Could you check a few things on this model? Use its own coordinates, in mm. Face numbers are marked on the shaded views. Give positions to 0.01 mm unless a question says otherwise; leave off trailing zeros. Order: outer loops, then holes, each group sorted by start corner. A loop starts at its lowest first (then second) coordinate and runs counter-clockwise, first axis right, second up. Notation, with made-up numbers: (18.5, -34) -> (53.5, -34) arc R26 ccw to (53.5, -9) -> close; hole circle Ø3 at (64, 29). An arc over 180 degrees is marked (long way). Write each question's results on one line, items separated by ' | '.
Autodesk Inventor part; units mm, degrees
ref_plane "YZ Plane" through (0, 0, 0) normal (1, 0, 0) x (0, 1, 0)
ref_plane "XZ Plane" through (0, 0, 0) normal (0, 1, 0) x (-1, 0, 0)
ref_plane "XY Plane" through (0, 0, 0) normal (0, 0, 1) x (1, 0, 0)
sketch "Sketch1" plane through (0, 0, 0) normal (0, 0, 1) x (1, 0, 0)
  circle A0 centre (0, 0) radius 30
  circle A1 centre (0, 0) radius 24.5
  dimension "d0" = 49
  dimension "d1" = 60
extrude "Extrusion1" add sketch "Sketch1" against normal blind 1.1
sketch "Sketch2" plane through (0, 0, 0) normal (0, 0, 1) x (1, 0, 0)
  line L0 (0, 0) -> (0, 30) construction
  circle A0 centre (0, 0) radius 30 construction
  line L1 (-1.7914, 26.2382) -> (1.7914, 26.2382)
  line L2 (1.7914, 26.2382) -> (1.7914, 29.0379)
  line L3 (1.7914, 29.0379) -> (-1.7914, 29.0379)
  line L4 (-1.7914, 29.0379) -> (-1.7914, 26.2382)
  line L5 (-1.7914, 26.2382) -> (1.7914, 29.0379) construction
  line L6 (1.7914, 26.2382) -> (-1.7914, 29.0379) construction
  point P0 (0, 27.6381)
extrude "Extrusion2" add sketch "Sketch2" along normal blind 1.7
pattern_circular "Circular Pattern1" count 15 over 360 about axis through (0, 0, -10) along (0, 0, 1) of "Extrusion2"
properties part number "LightRing"
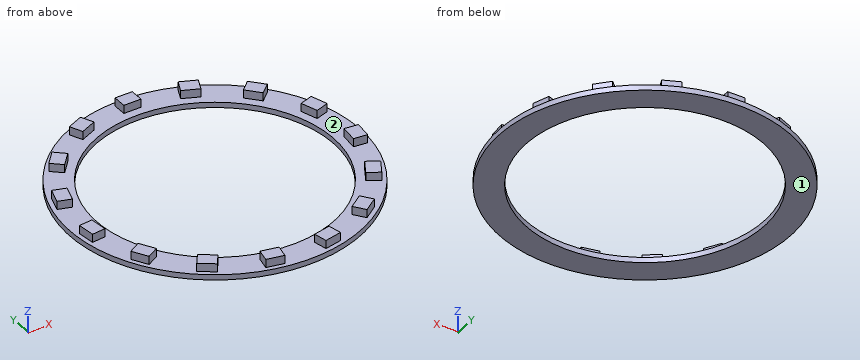
Q1. I'm going to push flat-ended pins straight in: pin 1 Ø6 at (x, y) = (-22, -22) entering from +Z; pin 2 Ø0.8 at (y, z) = (28, 1) entering from -X; pin 3 Ø1.4 at (y, z) = (27, 1) entering from +X. Where does each tip first touch, or does it pass through?
Here are the results:
pin 1: stops at z = 0 | pin 2: stops at x = -1.79 | pin 3: stops at x = 12.32
Q2. I need wall thicknesses on line 1 along Y through (x, z) = (0, -0.7); line 2 along X through (y, z) = (25.5, 0.2); line 3 along Y through (x, z) = (-0.5, 0.5). Which ranges of each line are inside material? Lowest first, please.
Here are the results:
line 1: y = -30 to -24.5, 24.5 to 30 | line 2: x = -13.31 to -9.39, 9.39 to 13.31 | line 3: y = 26.24 to 29.04
Q3. Suppose I cut it at B-B on x = 0. Please give me the cut outline in (y, z), and give its area (3 significant figures).
Here are the results:
outline: (-30, -1.1) -> (-24.5, -1.1) -> (-24.5, 0) -> (-30, 0) -> close; (24.5, -1.1) -> (30, -1.1) -> (30, 0) -> (29.04, 0) -> (29.04, 1.7) -> (26.24, 1.7) -> (26.24, 0) -> (24.5, 0) -> close | area: 16.9 mm²
Q4. Suppose I cut it at D-D on y = -17.5. Please give me the cut outline in (x, z).
Here are the results:
outline: (-24.37, -1.1) -> (-17.15, -1.1) -> (-17.15, 0) -> (-24.37, 0) -> close; (17.15, -1.1) -> (24.37, -1.1) -> (24.37, 0) -> (17.15, 0) -> close
Q5. Suppose I cut it at C-C on z = 0.7. State how many separate pieces and enclosed holes the cut face has, and give its area (3 significant figures).
Here are the results:
separate pieces: 15 | enclosed holes: 0 | area: 150 mm²
Q6. Thinking about a two-plate mould opening in X: for the marked faces 1 and 2, which applies, +X half, -X half, draft (parallel to the pull), parting line (faces both ways), or undercut?
Here are the results:
face 1: draft | face 2: undercut
Q7. Suppose I cut it at A-A on y = 0. Please give me the cut outline in (x, z).
Here are the results:
outline: (-30, -1.1) -> (-24.5, -1.1) -> (-24.5, 0) -> (-30, 0) -> close; (24.5, -1.1) -> (30, -1.1) -> (30, 0) -> (24.5, 0) -> close
